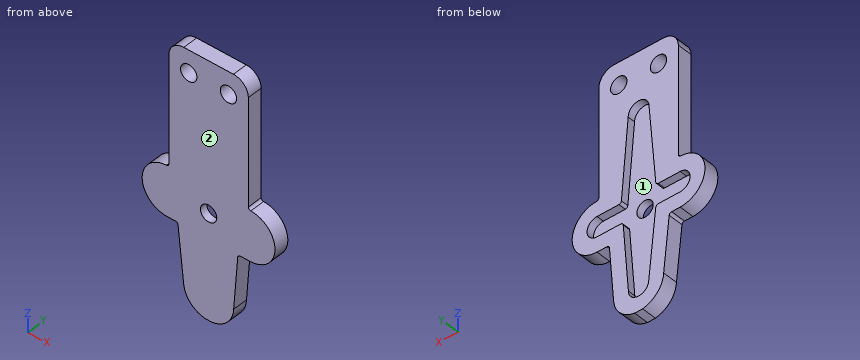
from build123d import *

# Parameters (mm, degrees)
SKETCH1_R               = 21
BOSS_EXTRUDE1_DEPTH     = 1.5
SKETCH5_W               = 16
SKETCH5_H               = 30
BOSS_EXTRUDE2_DEPTH     = 1.5
CUT_EXTRUDE1_DEPTH      = 1.5
CUT_EXTRUDE4_REACH      = 38.65
SKETCH4_R               = 1.65
CUT_EXTRUDE5_REACH      = 38.742
SKETCH6_R               = 1.65
CUT_EXTRUDE6_DEPTH      = 37.650375169
CUT_EXTRUDE6_DEPTH_BACK = 37.650375169
FILLET3_R               = 0.5
FILLET4_R               = 3


with BuildPart() as part:
    # Sketch1 → Boss-Extrude1 (new, symmetric)
    with BuildSketch(Plane(origin=(0, 0, 0), x_dir=(1, 0, 0), z_dir=(0, 1, 0))):
        with Locations(Location((0, 0, 0), (0, 0, 270))):
            Circle(SKETCH1_R)
    extrude(amount=BOSS_EXTRUDE1_DEPTH, both=True)

    # Sketch5 → Boss-Extrude2 (add, symmetric)
    with BuildSketch(Plane(origin=(0, 0, 0), x_dir=(1, 0, 0), z_dir=(0, 1, 0))):
        with Locations((0, -15)):
            Rectangle(SKETCH5_W, SKETCH5_H)
    extrude(amount=BOSS_EXTRUDE2_DEPTH, both=True)

    # Sketch2 → Cut-Extrude1 (cut)
    with BuildSketch(Plane(origin=(0, 1.5, 0), x_dir=(1, 0, 0), z_dir=(0, 1, 0))):
        with BuildLine():
            Line((-3.5, -2), (-2.1, -18.2))
            ThreePointArc((-2.1, -18.2), (0, -20.3), (2.1, -18.2))
            Line((2.1, -18.2), (3.5, -2))
            Line((3.5, -2), (8.375, -2))
            ThreePointArc((8.375, -2), (10.375, 0), (8.375, 2))
            Line((8.375, 2), (3.13, 2))
            Line((3.13, 2), (2.05, 16))
            ThreePointArc((2.05, 16), (0, 18.05), (-2.05, 16))
            Line((-2.05, 16), (-3.5, 2))
            Line((-3.5, 2), (-8.375, 2))
            ThreePointArc((-8.375, 2), (-10.375, 0), (-8.375, -2))
            Line((-8.375, -2), (-3.5, -2))
        make_face()
    extrude(amount=-CUT_EXTRUDE1_DEPTH, mode=Mode.SUBTRACT)

    # Sketch4 → Cut-Extrude4 (cut, up to next)
    with BuildSketch(Plane(origin=(0, 0, 0), x_dir=(1, 0, 0), z_dir=(0, 1, 0)), mode=Mode.PRIVATE) as cut_extrude4_sk1:
        with Locations(Location((0, 0, 0), (0, 0, 270))):
            Circle(SKETCH4_R)
    cut_extrude4_tool1 = extrude(cut_extrude4_sk1.sketch, amount=-CUT_EXTRUDE4_REACH, mode=Mode.PRIVATE) & part.part
    add(cut_extrude4_tool1.solids().sort_by_distance((0, 0, 0))[0], mode=Mode.SUBTRACT)

    # Sketch6 → Cut-Extrude5 (cut, up to next)
    with BuildSketch(Plane(origin=(0, 1.5, 0), x_dir=(1, 0, 0), z_dir=(0, 1, 0)), mode=Mode.PRIVATE) as cut_extrude5_sk1:
        with Locations(Location((4, -25.5, 0), (0, 0, 270))):
            Circle(SKETCH6_R)
    cut_extrude5_tool1 = extrude(cut_extrude5_sk1.sketch, amount=-CUT_EXTRUDE5_REACH, mode=Mode.PRIVATE) & part.part
    # Sketch6 → Cut-Extrude5 (cut, up to next)
    with BuildSketch(Plane(origin=(0, 1.5, 0), x_dir=(1, 0, 0), z_dir=(0, 1, 0)), mode=Mode.PRIVATE) as cut_extrude5_sk2:
        with Locations(Location((-4, -25.5, 0), (0, 0, 270))):
            Circle(SKETCH6_R)
    cut_extrude5_tool2 = extrude(cut_extrude5_sk2.sketch, amount=-CUT_EXTRUDE5_REACH, mode=Mode.PRIVATE) & part.part
    add(cut_extrude5_tool1.solids().sort_by_distance((4, 1.5, 25.5))[0], mode=Mode.SUBTRACT)
    add(cut_extrude5_tool2.solids().sort_by_distance((-4, 1.5, 25.5))[0], mode=Mode.SUBTRACT)

    # Sketch7 → Cut-Extrude6 (cut, two sides: drawn at the far end of the back side and taken through both)
    with BuildSketch(Plane(origin=(0, 0, 0), x_dir=(1, 0, 0), z_dir=(0, 1, 0)).offset(-CUT_EXTRUDE6_DEPTH_BACK)):
        with BuildLine():
            ThreePointArc((-0.811963461, 20.984296875), (-20.675312002, 3.678515137), (-8, -19.416487839))
            Line((-8, -19.416487839), (-8, -5))
            Line((-8, -5), (-8.375, -5))
            ThreePointArc((-8.375, -5), (-13.375, 0), (-8.375, 5))
            Line((-8.375, 5), (-6.205333354, 5))
            Line((-6.205333354, 5), (-5.046456013, 16.189160538))
            ThreePointArc((-5.046456013, 16.189160538), (-3.785314096, 19.342737979), (-0.811963461, 20.984296875))
        make_face()
        with BuildLine():
            ThreePointArc((8, -19.416487839), (20.675312002, 3.678515137), (0.811963461, 20.984296875))
            ThreePointArc((0.811963461, 20.984296875), (3.801185846, 19.324678355), (5.048028391, 16.141100531))
            Line((5.048028391, 16.141100531), (5.907484718, 5))
            Line((5.907484718, 5), (8.375, 5))
            ThreePointArc((8.375, 5), (13.375, 0), (8.375, -5))
            Line((8.375, -5), (8, -5))
            Line((8, -5), (8, -19.416487839))
        make_face()
    extrude(amount=CUT_EXTRUDE6_DEPTH + CUT_EXTRUDE6_DEPTH_BACK, mode=Mode.SUBTRACT)

    # Fillet3
    fillet3_edges = [part.edges().sort_by_distance(p)[0] for p in [
        (-8, 0, 5),
        (8, 0, 5),
        (-3.5, 0.75, -2),
        (3.5, 0.75, 2),
        (3.13, 0.75, -2),
        (-3.5, 0.75, 2),
        (-6.205333354, 0, -5),
        (5.907484718, 0, -5),
    ]]
    fillet(fillet3_edges, radius=FILLET3_R)

    # Fillet4
    fillet4_edges = [part.edges().sort_by_distance(p)[0] for p in [
        (8, 0, 30),
        (-8, 0, 30),
    ]]
    fillet(fillet4_edges, radius=FILLET4_R)


solid = part.part
Model file for the job. Use its own axes, mm. Face numbers are marked on the shaded views. Round coordinates to 2 decimals unless told otherwise and drop trailing zeros. Loops run counter-clockwise (first coordinate to the right, second up) from the corner with the lowest first, then second, coordinate; pieces in that order, holes last.
1. Band-saw the part on A-A, the plane z = 25.5. List the corners of the cut face in (x, y), and give its area (3 significant figures).
Check values:
outline: (-8, -1.5) - (-5.65, -1.5) - (-5.65, 1.5) - (-8, 1.5) - close; (-2.35, -1.5) - (2.35, -1.5) - (2.35, 1.5) - (-2.35, 1.5) - close; (5.65, -1.5) - (8, -1.5) - (8, 1.5) - (5.65, 1.5) - close
area: 28.2 mm2
2. Wall check: probe 1 along X at (y, z) = (0.85, 25.5); probe 2 along Y at (x, z) = (-1.5, 2.5); probe 3 along Z at (x, y) = (-9.75, 0.6). Give the ranges that are in metal, low to high.
Check values:
probe 1: x = -8 to -5.65, -2.35 to 2.35, 5.65 to 8
probe 2: y = -1.5 to 0
probe 3: z = -4.81 to -1.45, 1.45 to 4.81
3. Band-saw the part on B-B, the plane x = 0. List the corners of the cut face in (y, z).
Check values:
outline: (-1.5, -21) - (1.5, -21) - (1.5, -18.05) - (0, -18.05) - (0, -1.65) - (-1.5, -1.65) - close; (-1.5, 1.65) - (0, 1.65) - (0, 20.3) - (1.5, 20.3) - (1.5, 30) - (-1.5, 30) - close
4. Drop flat-ended pins along their axis: P1, Ø4.5, axis at x = 0, z = 0, coming from the +Y side; P2, Ø1, axis at y = 0, z = 22.5, coming from the +X side; P3, Ø0.8, axis at x = -5.5, y = 1, coming from the +Z side; P4, Ø1.5, axis at y = 0, z = 13.5, coming from the -X side. Give the stop position or say it passes through.
Check values:
P1: stops at y = 0
P2: stops at x = 8
P3: stops at z = 30
P4: stops at x = -8
5. Mould opens along X. For the marked faces 1 and 2 say: +X half, -X half, draft (parallel to the pull), parting line (faces both ways), or undercut.
Check values:
face 1: undercut
face 2: draft
6. Band-saw the part on C-C, the plane x = 9.5. List the corners of the cut face in (y, z), and give its area (3 significant figures).
Check values:
outline: (-1.5, -4.87) - (1.5, -4.87) - (1.5, -1.65) - (0, -1.65) - (0, 1.65) - (1.5, 1.65) - (1.5, 4.87) - (-1.5, 4.87) - close
area: 24.3 mm2
7. Band-saw the part on D-D, the plane z = 10. List the corners of the cut face in (x, y).
Check values:
outline: (-8, -1.5) - (8, -1.5) - (8, 1.5) - (2.81, 1.5) - (2.81, 0) - (-2.81, 0) - (-2.81, 1.5) - (-8, 1.5) - close
